Input: part model. Units: mm. Frame: model coordinates. A direction names the side the tool comes from. Round coordinates to 2 decimals unless told otherwise and drop trailing zeros. Loops run counter-clockwise (first coordinate to the right, second up) from the corner with the lowest first, then second, coordinate; pieces in that order, holes last. Notation, with made-up numbers: (3.5, 11.25) -> (51.5, 11.25) arc R4 cw to (51.5, 18.25) -> close; hole circle Ø6 at (37, 4.25). An arc over 180 degrees is marked (long way). Answer in a Markdown table with one row per item. Add a question column.
Q1. Section C-C, the plane x = -11. Output: boundary loops of the cut face in (y, z), and give its area (3 significant figures).
Q2. Section A-A, the plane x = -24. Output: boundary loops of the cut face in (y, z), and give its area (3 significant figures).
Q3. Section B-B, the plane z = 20. Output: boundary loops of the cut face in (x, y).
Q4. Section D-D, the plane y = 0.3. Output: boundary loops of the cut face in (x, z).
Q5. Ray query, L1, parallel to X at y = 1.2, z = 20; L2, parallel to Z at x = 21, y = 0.9; L3, parallel to Z at x = -24, y = 0.85. Return the intervals inside material, ascending. Write a range as from..to.
Q6. Reachability of faces 1 (the face through (26, 1, -31.8)), 2 (the face through (-20, 1, -31.8)), 3 (the face through (0, 2, 0)) from +Z, -Z, +X, -X, +Y, -Y: full face, straight path, thin tool, end or side. Return the list, or none.
Q7. Mould query, pull axis Z, two halves, no side actions, for faces 4 (the face through (0, 1, 34.3)), 5 (the face through (-25.08, 0.99, 18.82)), 6 (the face through (5, 1, -34.3)). Classes: pulls with the +Z half, pulls with the -Z half, needs draft (parallel to the pull), parting line crosses it, or undercut.
Q8. Pin query (flat end, axial travel): pin 1 (0.5 mm diameter, centred on x = 26, y = 1.5, fed in from -Z). Return the tip coordinate at first contact, or that it passes through.
Autodesk Inventor part; units mm, degrees
ref_plane "YZ Plane" through (0, 0, 0) normal (1, 0, 0) x (0, 1, 0)
ref_plane "XZ Plane" through (0, 0, 0) normal (0, 1, 0) x (-1, 0, 0)
ref_plane "XY Plane" through (0, 0, 0) normal (0, 0, 1) x (1, 0, 0)
sketch "Sketch1" plane through (0, 0, 0) normal (0, 1, 0) x (-1, 0, 0)
  line L0 (26.8759, 34.3) -> (-26.65, 34.3)
  line L1 (-25, -31.8) -> (-22, -34.3)
  line L2 (15, -31.8) -> (12, -34.3)
  line L3 (-25, -31.8) -> (-26.65, -31.8)
  line L4 (-22, -34.3) -> (12, -34.3)
  line L5 (-26.65, -31.8) -> (-26.65, 34.3)
  line L6 (25, -31.8) -> (26.8759, -30.2368)
  line L7 (25, -31.8) -> (15, -31.8)
  line L8 (26.8759, -30.2368) -> (26.8759, 34.3)
  line L9 (26.8759, 34.3) -> (-26.65, 34.3)
  line L10 (-26.65, -31.8) -> (-26.65, 34.3)
  line L11 (-26.65, -31.8) -> (-25, -31.8)
  line L12 (-25, -31.8) -> (-22, -34.3)
  line L13 (-22, -34.3) -> (12, -34.3)
  line L14 (12, -34.3) -> (15, -31.8)
  line L15 (15, -31.8) -> (25, -31.8)
  line L16 (25, -31.8) -> (26.8759, -30.2368)
  line L17 (26.8759, -30.2368) -> (26.8759, 34.3)
  point P0 (0, 0)
  point P1 (0, 0)
extrude "Extrusion1" add sketch "Sketch1" along normal blind 2
sketch "Sketch2" plane through (0, 2, 0) normal (0, 1, 0) x (1, 0, 0)
  line L0 (-26.8759, -34.3) -> (26.65, -34.3) construction
  line L1 (-24, -34.3) -> (-24, -20) construction
  circle A0 centre (-24, -20) radius 1.6
  line L2 (-0.1129, -34.3) -> (-0.1129, 34.3) construction
  line L3 (22, 34.3) -> (-12, 34.3) construction
  circle A1 centre (-24, -20) radius 1.6 construction
  circle A2 centre (23.7741, -20) radius 1.6
  point P0 (0, 0)
  dimension "d5" = 3.2
sketch "Sketch3" plane through (0, 2, 0) normal (0, 1, 0) x (1, 0, 0)
  circle A0 centre (-11, 31.8) radius 1.6 construction
  circle A1 centre (-11, 31.8) radius 1.6
  circle A2 centre (21, 31.8) radius 1.6
  line L0 (-18, -34.3) -> (-18, -38) construction
  line L1 (-18, -38) -> (-8, -38) construction
  line L2 (-8, -38) -> (-8, -34.3) construction
  line L3 (24, -36) -> (16, -36) construction
  line L4 (16, -36) -> (16, -34.3) construction
  line L5 (24, -34.3) -> (24, -36)
  line L6 (16, -36) -> (16, -34.3)
  line L7 (-8, -34.3) -> (-8, -38)
  line L8 (-18, -38) -> (-18, -34.3)
  line L9 (-18, -38) -> (-8, -38)
  line L10 (16, -36) -> (24, -36)
  line L11 (-18, -34.3) -> (-8, -34.3)
  line L12 (-26.8759, -34.3) -> (26.65, -34.3)
  line L13 (16, -34.3) -> (24, -34.3)
  line L14 (-26.8759, -34.3) -> (26.65, -34.3)
  line L15 (26.65, -34.3) -> (24, -34.3)
  line L16 (24, -34.3) -> (24, -36)
  line L17 (24, -36) -> (16, -36)
  line L18 (16, -34.3) -> (-8, -34.3)
  line L19 (-8, -34.3) -> (-8, -38)
  line L20 (-18, -38) -> (-18, -34.3)
  line L21 (-26.8759, 30.2368) -> (-25, 31.8)
  line L22 (-25, 31.8) -> (-26.8759, 30.2368)
  line L23 (-15, 31.8) -> (-12, 34.3)
  line L24 (-12, 34.3) -> (-15, 31.8)
  line L25 (-12, 34.3) -> (22, 34.3)
  line L26 (22, 34.3) -> (-12, 34.3)
  line L27 (22, 34.3) -> (25, 31.8)
  line L28 (25, 31.8) -> (22, 34.3)
  line L29 (25, 31.8) -> (26.65, 31.8)
  line L30 (26.65, 31.8) -> (26.65, -34.3)
  line L31 (-26.8759, -34.3) -> (26.65, -34.3)
  line L32 (-11, 31.8) -> (21, 31.8) construction
  line L33 (5, 31.8) -> (5, 0) construction
  point P0 (0, 0)
hole "Hole1" at (-24, 2, 20) at (23.7741, 2, 20) direction (0, -1, 0) diameter 3.2 depth 8 tip angle 118
hole "Hole2" at (-11, 2, -31.8) at (21, 2, -31.8) direction (0, -1, 0) diameter 3.2 depth 8 tip angle 118
properties part number "Arduino"
Answer block:
| question | item | result |
|---|---|---|
| 1 | outline | (0, -34.3) -> (2, -34.3) -> (2, -33.4) -> (0, -33.4) -> close; (0, -30.2) -> (2, -30.2) -> (2, 34.3) -> (0, 34.3) -> close |
| 1 | area | 131 mm^2 |
| 2 | outline | (0, -31.8) -> (2, -31.8) -> (2, 18.4) -> (0, 18.4) -> close; (0, 21.6) -> (2, 21.6) -> (2, 34.3) -> (0, 34.3) -> close |
| 2 | area | 126 mm^2 |
| 3 | outline | (-26.88, 0) -> (-25.6, 0) -> (-25.6, 2) -> (-26.88, 2) -> close; (-22.4, 0) -> (22.17, 0) -> (22.17, 2) -> (-22.4, 2) -> close; (25.37, 0) -> (26.65, 0) -> (26.65, 2) -> (25.37, 2) -> close |
| 4 | outline | (-26.88, -30.24) -> (-25, -31.8) -> (-15, -31.8) -> (-12, -34.3) -> (22, -34.3) -> (25, -31.8) -> (26.65, -31.8) -> (26.65, 34.3) -> (-26.88, 34.3) -> close; hole circle Ø3.2 at (-24, 20); hole circle Ø3.2 at (-11, -31.8); hole circle Ø3.2 at (21, -31.8); hole circle Ø3.2 at (23.77, 20) |
| 5 | L1 | -26.88..-25.6, -22.4..22.17, 25.37..26.65 |
| 5 | L2 | -34.3..-33.4, -30.2..34.3 |
| 5 | L3 | -31.8..18.4, 21.6..34.3 |
| 6 | face 1 | -Z, +X, +Y, -Y |
| 6 | face 2 | -Z, -X, +Y, -Y |
| 6 | face 3 | +Z, -Z, +X, -X, +Y |
| 7 | face 4 | pulls with the +Z half |
| 7 | face 5 | undercut |
| 7 | face 6 | pulls with the -Z half |
| 8 | pin 1 | z = -31.8 |
